```python
from build123d import *

# Parameters (mm, degrees)
SKETCH1_W               = 50
SKETCH1_H               = 200
BOSS_EXTRUDE1_DEPTH     = 20
SKETCH2_R               = 6
CUT_EXTRUDE1_DEPTH      = 84
FILLET1_R               = 10
SKETCH4_R               = 6
SKETCH4_R_2             = 1.5
CUT_EXTRUDE2_DEPTH      = 33
CUT_EXTRUDE3_DEPTH      = 1
CUT_EXTRUDE3_DEPTH_BACK = 53


with BuildPart() as part:
    # Sketch1 → Boss-Extrude1 (new body)
    with BuildSketch(Plane.XY):
        with Locations((25, -100)):
            Rectangle(SKETCH1_W, SKETCH1_H)
    extrude(amount=BOSS_EXTRUDE1_DEPTH)

    # Sketch2 → Cut-Extrude1 (cut)
    with BuildSketch(Plane.XY.offset(20)):
        with Locations((25, -185)):
            Circle(SKETCH2_R)
        with Locations((25, -15)):
            Circle(SKETCH2_R)
    extrude(amount=-CUT_EXTRUDE1_DEPTH, mode=Mode.SUBTRACT)

    # Fillet1
    fillet1_edges = [part.edges().sort_by_distance(p)[0] for p in [
        (0, 0, 10),
        (50, 0, 10),
        (50, -200, 10),
        (0, -200, 10),
    ]]
    fillet(fillet1_edges, radius=FILLET1_R)

    # Sketch4 → Cut-Extrude2 (cut)
    with BuildSketch(Plane.XY.offset(20)):
        Polygon((31.2, -8.8), (25, -8.8), (18.8, -8.8), (18.8, -31.3), (25, -31.3), (31.2, -31.3), align=None)
        with Locations((25, -15)):
            Circle(SKETCH4_R, mode=Mode.SUBTRACT)
        with Locations((25, -33.7)):
            Circle(SKETCH4_R_2)
        with Locations((25, -6.4)):
            Circle(SKETCH4_R_2)
    extrude(amount=-CUT_EXTRUDE2_DEPTH, mode=Mode.SUBTRACT)

    # Sketch5 → Cut-Extrude3 (cut, two sides)
    with BuildSketch(Plane.XY.offset(20)) as cut_extrude3_sk:
        with BuildLine():
            ThreePointArc((49.469995195, -179.879518072), (49.867145794, -182.426080796), (50, -185))
            Line((50, -185), (50, -15))
            ThreePointArc((50, -15), (49.867145794, -17.573919204), (49.469995195, -20.120481928))
            ThreePointArc((49.469995195, -20.120481928), (41.201920232, -100), (49.469995195, -179.879518072))
        make_face()
        with BuildLine():
            ThreePointArc((0.530004805, -20.120481928), (0.132854206, -17.573919204), (0, -15))
            Line((0, -15), (0, -185))
            ThreePointArc((0, -185), (0.132854206, -182.426080796), (0.530004805, -179.879518072))
            ThreePointArc((0.530004805, -179.879518072), (8.798079768, -100), (0.530004805, -20.120481928))
        make_face()
    extrude(amount=CUT_EXTRUDE3_DEPTH, mode=Mode.SUBTRACT)
    extrude(cut_extrude3_sk.sketch, amount=-CUT_EXTRUDE3_DEPTH_BACK, mode=Mode.SUBTRACT)


solid = part.part
```
Work out the finished part from the listing and answer in its coordinate system (mm). A direction names the side the tool comes from. Round coordinates to 2 decimals unless told otherwise and drop trailing zeros. Write each loop counter-clockwise with the first axis right and the second up, starting at its lowest first coordinate (ties: lowest second). Pieces come first, ordered by that corner, then holes.
1) Flat-ended cylindrical pins translate along their axes: P1, Ø12, axis at y = -45.5, z = 12, coming from the +X side; P2, Ø10, axis at y = -124.5, z = 11, coming from the -X side; P3, Ø11, axis at x = 25, y = -185, coming from the +Z side; P4, Ø6, axis at x = 45, z = 17.5, coming from the -Y side. Find the tip coordinate at first contact, or state that the pin passes through.
2) A cutting plane is placed at A-A on z = 2. Determine the outline of the cut face in (x, y), and give its area (3 significant figures).
3) Consider probe 1 along Y at (x, z) = (25, 11.5); probe 2 along Y at (x, z) = (24, 3.5); probe 3 along X at (y, z) = (-180.5, 3.25). Determine where each line is inside the solid, lowest interval first.
4) Determine the mould class of faces 1 (the face through (25, -99, 20)), 2 (the face through (25, -8.8, 10)), 3 (the face through (2.85, -3.01, 10.14)) for opening direction Y: pulls with the +Y half, pulls with the -Y half, needs draft (parallel to the pull), parting line crosses it, or undercut.
5) A cutting plane is placed at C-C on y = -84. Determine the outline of the cut face in (x, z).
6) A cutting plane is placed at B-B on x = 43. Determine the outline of the cut face in (y, z).
7) Which of the six approach directions +Z, -Z, +X, -X, +Y, -Y give full straight-line access (tool end or side, diameter ignored) to faces 4 (the face through (0.137, -17.61, 10.14)), 5 (the face through (18.8, -20, 10)), 6 (the face through (49.87, -17.54, 10.14))?
Entries:
1. P1: stops at x = 45.92
1. P2: stops at x = 7.68
1. P3: passes through
1. P4: stops at y = -199.8
2. outline: (0, -190) arc R10 ccw to (10, -200) - (40, -200) arc R10 ccw to (50, -190) - (50, -185) arc R25 ccw to (49.47, -179.88) arc R390 cw to (49.47, -20.12) arc R25 ccw to (50, -15) - (50, -10) arc R10 ccw to (40, 0) - (10, 0) arc R10 ccw to (0, -10) - (0, -15) arc R25 ccw to (0.53, -20.12) arc R390 cw to (0.53, -179.88) arc R25 ccw to (0, -185) - close; hole (18.8, -31.3) - (31.2, -31.3) - (31.2, -8.8) - (18.8, -8.8) - close; hole circle Ø12 at (25, -185); hole circle Ø3 at (25, -33.7); hole circle Ø3 at (25, -6.4)
2. area: 7,570 mm2
3. probe 1: y = -200 to -191, -179 to -35.2, -32.2 to -31.3, -8.8 to -7.9, -4.9 to 0
3. probe 2: y = -200 to -190.92, -179.08 to -34.82, -32.58 to -31.3, -8.8 to -7.52, -5.28 to 0
3. probe 3: x = 0.41 to 21.03, 28.97 to 49.59
4. face 1: needs draft
4. face 2: undercut
4. face 3: pulls with the +Y half
5. outline: (8.47, 0) - (41.53, 0) - (41.53, 20) - (8.47, 20) - close
6. outline: (-199.54, 0) - (-137.41, 0) - (-137.41, 20) - (-199.54, 20) - close; (-62.59, 0) - (-0.46, 0) - (-0.46, 20) - (-62.59, 20) - close
7. face 4: +Z, -Z, -X
7. face 5: +Z, -Z
7. face 6: +Z, -Z, +X
